The listing builds one solid part. Answer for the finished solid, in the listing's coordinates (mm). Round coordinates to 2 decimals unless told otherwise and drop trailing zeros. Loops run counter-clockwise (first coordinate to the right, second up) from the corner with the lowest first, then second, coordinate; pieces in that order, holes last. Notation, with made-up numbers: M 89,80 L 107,80 A6 ccw 107,86 Z; hole C 59,-25.75 d2. An arc over 180 degrees is marked long. Answer as a JSON object with one key per item and string values.
```python
from build123d import *

# Parameters (mm, degrees)
F0_W      = 508
F0_H      = 254
F1_DEPTH  = 38.1
F2_R      = 12.7
F1_FACE_W = 482.6
F1_FACE_H = 228.6
F3_DEPTH  = 2.54


with BuildPart() as f1:
    # F0 (on Front) → F1 (new body)
    with BuildSketch(Plane.XZ):
        Rectangle(F0_W, F0_H)
    extrude(amount=F1_DEPTH)

    # F2
    f2_edges = [f1.edges().sort_by_distance(p)[0] for p in [
        (254, -38.1, 0),
        (0, -38.1, 127),
        (-254, -38.1, 0),
        (0, -38.1, -127),
        (-254, -19.05, 127),
        (254, -19.05, 127),
        (254, -19.05, -127),
        (-254, -19.05, -127),
    ]]
    fillet(f2_edges, radius=F2_R)

    # F1_face (on face) → F3 (cut)
    with BuildSketch(Plane.XZ.offset(38.1)):
        Rectangle(F1_FACE_W, F1_FACE_H)
    extrude(amount=-F3_DEPTH, mode=Mode.SUBTRACT)


solid = f1.part
```
Item 1: Determine the mould class of faces 1 (the face through (-250.38, -34.28, 1.6)), 2 (the face through (250.18, -12.88, -123.38)), 3 (the face through (-3, -35.56, 2)) for opening direction Z: released by +Z, released by -Z, zero draft, split by the parting line, or undercut.
Values follow:
{"face 1": "zero draft", "face 2": "released by -Z", "face 3": "undercut"}
Item 2: Flat-ended cylindrical pins translate along their axes: P1, Ø1, axis at x = 161, z = 18, coming from the -Y side; P2, Ø0.8, axis at y = -37, z = 49, coming from the +X side; P3, Ø1.3, axis at y = -37, z = -37, coming from the -X side. Find the tip coordinate at first contact, or state that the pin passes through.
Values follow:
{"P1": "y = -35.56", "P2": "x = 247.29", "P3": "x = -247.73"}
Item 3: The part is cut by section B-B (z = 12). Give the vertices of the cut face in (x, y).
Values follow:
{"outline": "M -254,-25.4 A12.7 ccw -241.3,-38.1 L -241.3,-35.56 L 241.3,-35.56 L 241.3,-38.1 A12.7 ccw 254,-25.4 L 254,0 L -254,0 Z"}
Item 4: Straight lines are drawn through the part: line 1 (Y direction, x = -87, z = -22.5); line 2 (X direction, y = -36, z = -37) (3 decimals); line 3 (Z direction, x = 231.5, y = -25.5). For each, find the intervals that lie inside material, in ascending order.
Values follow:
{"line 1": "-35.56 to 0", "line 2": "-248.295 to -241.3, 241.3 to 248.295", "line 3": "-127 to 127"}
Item 5: The part is cut by section A-A (x = 47.5). Give the vertices of the cut face in (y, z).
Values follow:
{"outline": "M -38.1,-114.3 A12.7 ccw -25.4,-127 L 0,-127 L 0,127 L -25.4,127 A12.7 ccw -38.1,114.3 L -35.56,114.3 L -35.56,-114.3 Z"}
